Verification items for the finished model (mm, model axes). A direction names the side the tool comes from. Give positions to 0.01 mm unless a question says otherwise; leave off trailing zeros. Order: outer loops, then holes, each group sorted by start corner. A loop starts at its lowest first (then second) coordinate and runs counter-clockwise, first axis right, second up.
(1) Gauge pin test, flat ends, axial feed: pin 1 (1.5 mm diameter, centred on x = 10, y = -5, fed in from -Z); pin 2 (2 mm diameter, centred on x = 28.5, y = 1.5, fed in from +Z); pin 3 (4 mm diameter, centred on x = 22.5, y = 3.5, fed in from +Z). Record the tip position at first contact, or that the pin passes through.
(2) Mould release check, pull along X, two halves, no side actions. Record for faces 1 (the face through (44.3, -3, -4)), 2 (the face through (0.35, -5, -3.83)), 3 (the face through (5.49, 3.31, -6.37)): pulls with the +X half, pulls with the -X half, needs draft (parallel to the pull), parting line crosses it, or undercut.
(3) Scan lines: L1, parallel to Z at x = 22, y = 0 (3 decimals); L2, parallel to X at y = -0.25, z = -6.25; L3, parallel to Y at x = 33, z = 0.5. Record each from-to range of solid material in increasing order.
(4) Sectioned sample at A-A on x = 27.5. Record the cut outline in (y, z) (3 decimals), plus the area to 3 significant figures.
(5) Access from +Z, -Z, +X, -X, +Y, -Y to the whole of each face (thin tool, end or side, straight path). Record for faces 4 (the face through (44.65, -5, -3.83)), 5 (the face through (39.49, 3.31, -6.37)), 6 (the face through (2.718, -7.493, 0.33)).
```python
from build123d import *

# Parameters (mm, degrees)
ZKOSEN_1_SIZE = 0.5


with BuildPart() as part:
    # Skica1 → Rotovat1 (revolve)
    with BuildSketch(Plane.XY):
        Polygon((0, 4.3), (0, 4.175), (45, 4.175), (45, 4.3), (44.3, 4.3), (44.3, 6.3), (45, 6.3), (45, 7.5), (40, 7.5), (40, 7.18), (39, 7.18), (39, 7.5), (6, 7.5), (6, 7.18), (5, 7.18), (5, 7.5), (0, 7.5), (0, 6.3), (0.7, 6.3), (0.7, 4.3), align=None)
    revolve(axis=Axis((0, 0, 0), (1, 0, 0)))

    # Zkosení1
    zkosen_1_edges = [part.edges().sort_by_distance(p)[0] for p in [
        (0, -7.5, 0),
        (45, -7.5, 0),
    ]]
    chamfer(zkosen_1_edges, length=ZKOSEN_1_SIZE)


solid = part.part
```
Ans:
1. pin 1: stops at z = -6.18
1. pin 2: stops at z = 7.48
1. pin 3: stops at z = 7.35
2. face 1: pulls with the +X half
2. face 2: needs draft
2. face 3: undercut
3. L1: z = -7.5 to -4.175, 4.175 to 7.5
3. L2: x = 0.7 to 44.3
3. L3: y = -7.48 to -4.14, 4.14 to 7.48
4. outline: circle Ø15 at (0, 0); hole circle Ø8.35 at (0, 0)
4. area: 122 mm2
5. face 4: +X
5. face 5: none
5. face 6: +X, -X
